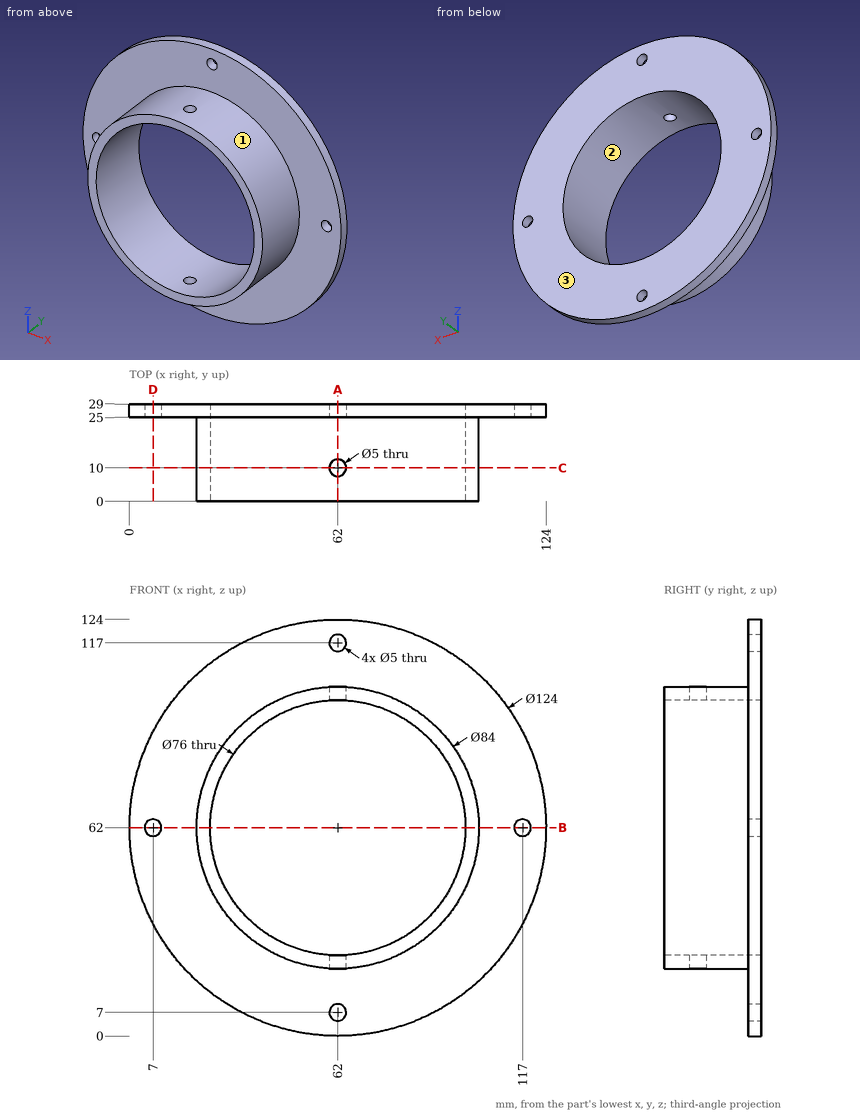
Geometry check sheet. Reference: drawing and pictorial views, mm from the part's lowest x, y, z. Round coordinates to 2 decimals unless told otherwise and drop trailing zeros. Order: outer loops, then holes, each group sorted by start corner. A loop starts at its lowest first (then second) coordinate and runs counter-clockwise, first axis right, second up. Notation, with made-up numbers: M 82,59.5 L 119,59.5 A9 cw 119,70.5 Z; hole C -2,2.25 d8. An arc over 180 degrees is marked long. Answer in a Markdown table with one row per item.
(1) Draft check along Z on the marked faces 1, 2 and 3. Enter one of: released by +Z, released by -Z, zero draft, split by the parting line, or undercut.
Responses:
| item | result |
|---|---|
| face 1 | split by the parting line |
| face 2 | undercut |
| face 3 | zero draft |
(2) Scan lines: probe 1 along X at (y, z) = (26.15, 62); probe 2 along Z at (x, y) = (43.5, 17); probe 3 along Y at (x, z) = (27, 102). Record each from-to range of solid material in increasing order. Write a range as from..to.
Responses:
| item | result |
|---|---|
| probe 1 | x = 0..4.5, 9.5..24, 100..114.5, 119.5..124 |
| probe 2 | z = 24.29..28.81, 95.19..99.71 |
| probe 3 | y = 25..29 |
(3) Go/stop test with flat-tipped pins: P1, Ø4.5, axis at x = 7, z = 62, coming from the +Y side; P2, Ø6, axis at x = 62, z = 7, coming from the -Y side; P3, Ø8, axis at x = 62, y = 10, coming from the +Z side; P4, Ø8, axis at x = 86, y = 10.5, coming from the -Z side. Record where each tip stops, or that it passes through.
Responses:
| item | result |
|---|---|
| P1 | passes through |
| P2 | stops at y = 25 |
| P3 | stops at z = 104 |
| P4 | stops at z = 25.07 |
(4) Sectioned sample at A-A, the plane x = 62. Record the cut outline in (y, z).
Responses:
| item | result |
|---|---|
| outline | M 0,20 L 7.5,20 L 7.5,24 L 0,24 Z; M 0,100 L 7.5,100 L 7.5,104 L 0,104 Z; M 12.5,20 L 25,20 L 25,9.5 L 29,9.5 L 29,24 L 12.5,24 Z; M 12.5,100 L 29,100 L 29,114.5 L 25,114.5 L 25,104 L 12.5,104 Z; M 25,0 L 29,0 L 29,4.5 L 25,4.5 Z; M 25,119.5 L 29,119.5 L 29,124 L 25,124 Z |
(5) Sectioned sample at C-C, the plane y = 10. Record the cut outline in (x, z).
Responses:
| item | result |
|---|---|
| outline | M 59.5,20.07 L 59.5,24.08 A38 cw 59.5,99.92 L 59.5,103.93 A42 ccw Z; M 64.5,20.07 A42 ccw 64.5,103.93 L 64.5,99.92 A38 cw 64.5,24.08 Z |
(6) Sectioned sample at B-B, the plane z = 62. Record the cut outline in (x, y), and give its area (3 significant figures).
Responses:
| item | result |
|---|---|
| outline | M 0,25 L 4.5,25 L 4.5,29 L 0,29 Z; M 9.5,25 L 20,25 L 20,0 L 24,0 L 24,29 L 9.5,29 Z; M 100,0 L 104,0 L 104,25 L 114.5,25 L 114.5,29 L 100,29 Z; M 119.5,25 L 124,25 L 124,29 L 119.5,29 Z |
| area | 352 mm² |
(7) Sectioned sample at D-D, the plane x = 7. Record the cut outline in (y, z).
Responses:
| item | result |
|---|---|
| outline | M 25,33.38 L 29,33.38 L 29,59.5 L 25,59.5 Z; M 25,64.5 L 29,64.5 L 29,90.62 L 25,90.62 Z |
